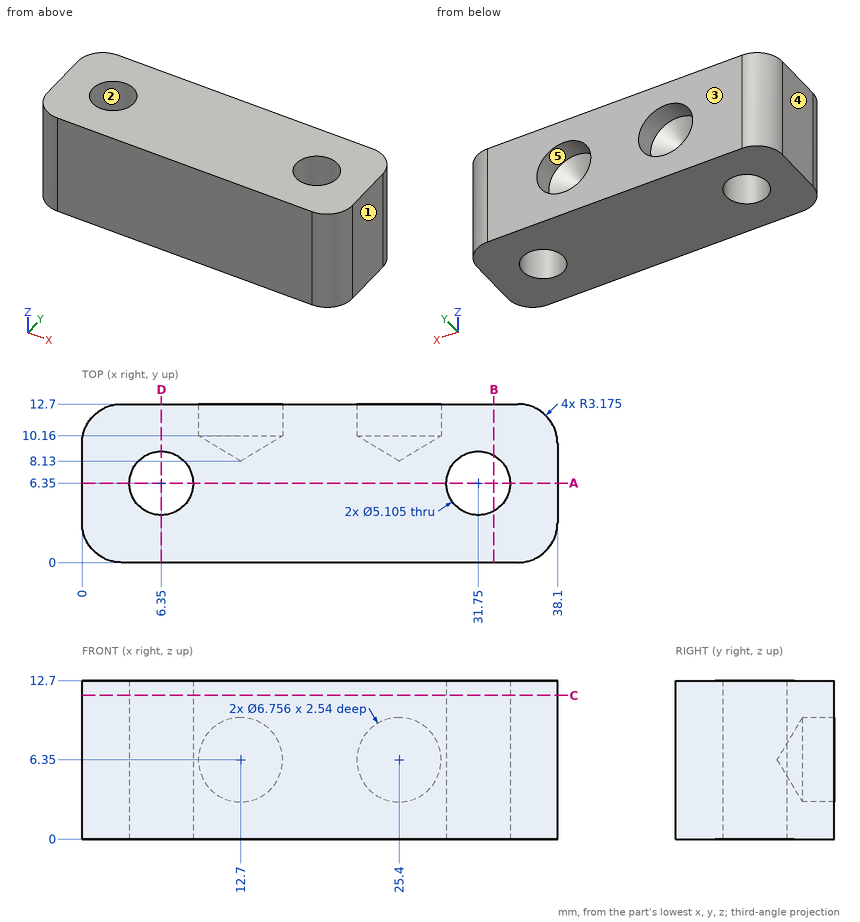
Geometry check sheet. Reference: drawing and pictorial views, mm from the part's lowest x, y, z. A direction names the side the tool comes from. Round coordinates to 2 decimals unless told otherwise and drop trailing zeros. Order: outer loops, then holes, each group sorted by start corner. A loop starts at its lowest first (then second) coordinate and runs counter-clockwise, first axis right, second up. Notation, with made-up numbers: (55, 55) - (103, 55) arc R27 ccw to (103, 93) - close; hole circle Ø7 at (-24, -34.75). An arc over 180 degrees is marked (long way). Use a Markdown table: item, result. Add a question column.
1) Section check C-C (z = 11.5). Count the separate pieces of the cut face and the enclosed holes in it, then the cut area to 3 significant figures.
2) Gauge pin test, flat end, axial feed: P1, Ø1.5, axis at x = 33, y = 7, coming from the -Z side. Record the tip position at first contact, or that the pin passes through.
3) Section check B-B (x = 33). Record the cut outline in (y, z) (1 decimal), then the cut area to 3 significant figures.
4) Set-up check for the marked faces 4 and 5: record each of +Z, -Z, +X, -X, +Y, -Y from which the full face is reachable in a straight line by a thin tool's end or side.
5) Section check A-A (y = 6.35). Record the cut outline in (x, z).
6) Section check D-D (x = 6.35). Record the cut outline in (y, z).
7) Mould release check, pull along X, two halves, no side actions. Record for the marked faces 1, 2 and 3: released by +X, released by -X, zero draft, split by the parting line, or undercut.
8) Thickness scan on line 1 along X through (y, z) = (6.25, 5); line 2 along X through (y, z) = (5.75, 2.5); line 3 along Z through (x, y) = (25.4, 11.45). Record the ranges inside material, lowest first.
Established:
| question | item | result |
|---|---|---|
| 1 | separate pieces | 1 |
| 1 | enclosed holes | 2 |
| 1 | area | 434 mm2 |
| 2 | P1 | through |
| 3 | outline | (0, 0) - (4.1, 0) - (4.1, 12.7) - (0, 12.7) - close; (8.6, 0) - (12.7, 0) - (12.7, 12.7) - (8.6, 12.7) - close |
| 3 | area | 105 mm2 |
| 4 | face 4 | +Z, -Z, -X, +Y, -Y |
| 4 | face 5 | +Y |
| 5 | outline | (0, 0) - (3.8, 0) - (3.8, 12.7) - (0, 12.7) - close; (8.9, 0) - (29.2, 0) - (29.2, 12.7) - (8.9, 12.7) - close; (34.3, 0) - (38.1, 0) - (38.1, 12.7) - (34.3, 12.7) - close |
| 6 | outline | (0, 0) - (3.8, 0) - (3.8, 12.7) - (0, 12.7) - close; (8.9, 0) - (12.7, 0) - (12.7, 12.7) - (8.9, 12.7) - close |
| 7 | face 1 | released by +X |
| 7 | face 2 | undercut |
| 7 | face 3 | zero draft |
| 8 | line 1 | 0 to 3.8, 8.9 to 29.2, 34.3 to 38.1 |
| 8 | line 2 | 0 to 3.87, 8.83 to 29.27, 34.23 to 38.1 |
| 8 | line 3 | 0 to 2.97, 9.73 to 12.7 |
